Check sheet for the modelled part. Datum: model origin and axes. Units: mm. Give positions to 0.01 mm unless a question says otherwise; leave off trailing zeros. Write each loop counter-clockwise with the first axis right and the second up, starting at its lowest first coordinate (ties: lowest second). Pieces come first, ordered by that corner, then holes. Notation, with made-up numbers: M -13,61 L 37,61 A26 ccw 37,81 Z; hole C 22.25,-7 d11. An arc over 180 degrees is marked long. Write item = value, one per line. Start each with the question number.
1) Go/stop test with a flat-tipped pin: pin 1 (1 mm diameter, centred on x = 43.5, z = -27, fed in from +Y). Record where the tip stops, or that it passes through.
2) Scan lines: line 1 along Z through (x, y) = (9, 29.5); line 2 along Y through (x, z) = (30, -30); line 3 along Z through (x, y) = (21, 25). Record each from-to range of solid material in increasing order. Write a range as [from, to].
3) Cross-section at A-A, the plane x = -19.5. Record the cut outline in (y, z), plus the area to 3 significant figures.
4) Cross-section at C-C, the plane z = -36. Record the cut outline in (x, y).
5) Cross-section at B-B, the plane y = 24.5. Record the cut outline in (x, z), plus the area to 3 significant figures.
Autodesk Inventor part; units mm, degrees
ref_plane "YZ Plane" through (0, 0, 0) normal (1, 0, 0) x (0, 1, 0)
ref_plane "XZ Plane" through (0, 0, 0) normal (0, 1, 0) x (-1, 0, 0)
ref_plane "XY Plane" through (0, 0, 0) normal (0, 0, 1) x (1, 0, 0)
sketch "Sketch1" plane through (0, 0, 0) normal (1, 0, 0) x (0, 1, 0)
  line L0 (0, 0) -> (38.1, 0)
  line L1 (38.1, 0) -> (38.1, -19.05)
  line L2 (19.05, -38.1) -> (0, -38.1)
  line L3 (0, -38.1) -> (0, 0)
  arc A0 (38.1, -19.05) -> (19.05, -38.1) centre (38.1, -38.1) ccw
  dimension "d0" = 38.1
  dimension "d1" = 38.1
  dimension "d2" = 38.1
  dimension "d5" = 38.1
  dimension "d6" = 38.1
extrude "Extrusion1" add sketch "Sketch1" along normal mid plane 152.4
properties part number "chuckFor_0_75_inchQuarterRound"
Reply:
q1.pin_1 = 22.99
q2.line_1 = [-21.1, 0]
q2.line_2 = [0, 20.86]
q2.line_3 = [-24.27, 0]
q3.outline = M 0,-38.1 L 19.05,-38.1 A19.05 cw 38.1,-19.05 L 38.1,0 L 0,0 Z
q3.area = 1,170 mm2
q4.outline = M -76.2,0 L 76.2,0 L 76.2,19.17 L -76.2,19.17 Z
q5.outline = M -76.2,-24.76 L 76.2,-24.76 L 76.2,0 L -76.2,0 Z
q5.area = 3,770 mm2
